Design review of the part built by this model. Coordinates are the model's own, in mm. Face numbers are marked on the shaded views. A direction names the side the tool comes from. Give positions to 0.01 mm unless a question says otherwise; leave off trailing zeros. Loops run counter-clockwise (first coordinate to the right, second up) from the corner with the lowest first, then second, coordinate; pieces in that order, holes last. Notation, with made-up numbers: M 65.25,-4 L 95.25,-4 A30 cw 95.25,32 Z; hole C -5.5,-2.75 d11. An arc over 180 degrees is marked long. Use a Markdown table: item, result. Add a question column.
(1) For the marked faces 4, 5 and 6, list the 3-axis set-ups (+Z, -Z, +X, -X, +Y, -Y) from which the entire face can be reached by the end or side of a thin tool; tool diameter is ignored.
(2) Add section A-A, the plane z = 27.5. Give the boundary of the cut face in (x, y).
(3) Add section C-C, the plane x = 86.5. Give the boundary of the cut face in (y, z).
(4) Add section D-D, the plane z = 16. Give the boundary of the cut face in (x, y).
(5) Insertion check: pin 1 Ø5 at (y, z) = (10, 14) entering from -X; pin 2 Ø10 at (x, z) = (24.5, 18) entering from -Y; pin 3 Ø5 at (x, z) = (34.92, 23.24) entering from +Y; pin 4 Ø1.9 at (y, z) = (11, 8) entering from +X. Each pin has a flat end and moves straight along its axis. Give the tip position at first contact, or say it passes through.
(6) For probe 1 along X at (y, z) = (7, 2); probe 2 along X at (y, z) = (9, 18.5); probe 3 along X at (y, z) = (7.5, 7.5), list the stretches that pass through material, from the lowest coordinate up.
(7) Add section B-B, the plane y = 9.5. State how many separate pieces and enclosed holes the cut face has, then the cut area to 3 significant figures.
(8) Draft analysis for pull direction Z (two halves, no side actions). For the marked faces 1, 2 and 3, state which applies: pulls with the +Z half, pulls with the -Z half, needs draft (parallel to the pull), parting line crosses it, or undercut.
```python
from build123d import *

# Parameters (mm, degrees)
F0_W      = 12.7
F0_H      = 31.75
F1_DEPTH  = 139.7
F2_W      = 12.7
F2_H      = 6.35
F2_W_2    = 6.35
F3_DEPTH  = 31.751
F4_R      = 2.159
F5_DEPTH  = 25.4
F6_R      = 2.159
F7_DEPTH  = 25.4
F8_W      = 50.8
F8_H      = 19.05
F9_DEPTH  = 6.35
F10_W     = 6.35
F10_H     = 19.05
F11_DEPTH = 6.35
F12_R     = 3.17499


# Not quite as in the source:
# - a fillet or chamfer is up to 0.001 mm smaller than in the source, because OpenCascade refuses the exact size


with BuildPart() as f1:
    # F0 (on Right) → F1 (new body)
    with BuildSketch(Plane.YZ):
        with Locations((6.35, 15.875)):
            Rectangle(F0_W, F0_H)
    extrude(amount=F1_DEPTH)

    # F2 (on face) → F3 (cut, through all)
    with BuildSketch(Plane.XY.offset(31.75)):
        with Locations((6.35, 9.525)):
            Rectangle(F2_W, F2_H)
        with Locations((34.925, 9.525)):
            Rectangle(F2_W_2, F2_H)
        with Locations((104.775, 9.525)):
            Rectangle(F2_W_2, F2_H)
        with Locations((133.35, 9.525)):
            Rectangle(F2_W, F2_H)
    extrude(amount=-F3_DEPTH, mode=Mode.SUBTRACT)

    # F4 (on face) → F5 (cut)
    with BuildSketch(Plane.XZ):
        with Locations((6.3445889391, 23.241)):
            Circle(F4_R)
        with Locations((6.3445889391, 8.509)):
            Circle(F4_R)
        with BuildLine():
            ThreePointArc((135.5180395808, 8.509), (133.3590395808, 10.668), (131.2000395808, 8.509))
            ThreePointArc((131.2000395808, 8.509), (133.3590395808, 6.35), (135.5180395808, 8.509))
        make_face()
        with BuildLine():
            ThreePointArc((135.5180395808, 23.241), (133.3590395808, 25.4), (131.2000395808, 23.241))
            ThreePointArc((131.2000395808, 23.241), (133.3590395808, 21.082), (135.5180395808, 23.241))
        make_face()
    extrude(amount=-F5_DEPTH, mode=Mode.SUBTRACT)

    # F6 (on face) → F7 (cut)
    with BuildSketch(Plane.XZ):
        with Locations((34.9172241986, 23.241)):
            Circle(F6_R)
        with Locations((34.9172241986, 8.509)):
            Circle(F6_R)
        with Locations((104.6765521169, 8.509)):
            Circle(F6_R)
        with Locations((104.6765521169, 23.241)):
            Circle(F6_R)
    extrude(amount=-F7_DEPTH, mode=Mode.SUBTRACT)

    # F8 (on face) → F9 (cut)
    with BuildSketch(Plane(origin=(0, 12.7, 0), x_dir=(-1, 0, 0), z_dir=(0, 1, 0))):
        with Locations((-69.85, 15.875)):
            Rectangle(F8_W, F8_H)
    extrude(amount=-F9_DEPTH, mode=Mode.SUBTRACT)

    # F10 (on face) → F11 (cut)
    with BuildSketch(Plane(origin=(0, 12.7, 0), x_dir=(-1, 0, 0), z_dir=(0, 1, 0))):
        with Locations((-22.225, 15.875)):
            Rectangle(F10_W, F10_H)
        with Locations((-117.475, 15.875)):
            Rectangle(F10_W, F10_H)
    extrude(amount=-F11_DEPTH, mode=Mode.SUBTRACT)

    # F12 (radius 3.175 in the source; OpenCascade refuses exactly that, so slightly less here)
    f12_edges = [f1.edges().sort_by_distance(p)[0] for p in [
        (19.05, 9.525, 6.35),
        (25.4, 9.525, 6.35),
        (19.05, 9.525, 25.4),
        (25.4, 9.525, 25.4),
        (44.45, 9.525, 6.35),
        (95.25, 9.525, 6.35),
        (95.25, 9.525, 25.4),
        (44.45, 9.525, 25.4),
        (120.65, 9.525, 6.35),
        (120.65, 9.525, 25.4),
        (114.3, 9.525, 25.4),
        (114.3, 9.525, 6.35),
    ]]
    fillet(f12_edges, radius=F12_R)


solid = f1.part
```
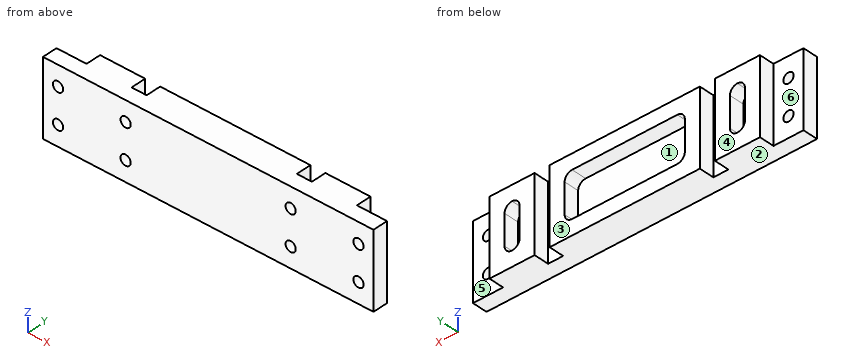
Established:
| question | item | result |
|---|---|---|
| 1 | face 4 | +Z, -Z, +X, -X, +Y |
| 1 | face 5 | +Z, -Z, +X, +Y |
| 1 | face 6 | +Z, -Z, -X, +Y |
| 2 | outline | M 0,0 L 139.7,0 L 139.7,6.35 L 127,6.35 L 127,12.7 L 107.95,12.7 L 107.95,6.35 L 101.6,6.35 L 101.6,12.7 L 38.1,12.7 L 38.1,6.35 L 31.75,6.35 L 31.75,12.7 L 12.7,12.7 L 12.7,6.35 L 0,6.35 Z |
| 3 | outline | M 0,0 L 12.7,0 L 12.7,6.35 L 6.35,6.35 L 6.35,25.4 L 12.7,25.4 L 12.7,31.75 L 0,31.75 Z |
| 4 | outline | M 0,0 L 139.7,0 L 139.7,6.35 L 127,6.35 L 127,12.7 L 120.65,12.7 L 120.65,6.35 L 114.3,6.35 L 114.3,12.7 L 107.95,12.7 L 107.95,6.35 L 101.6,6.35 L 101.6,12.7 L 95.25,12.7 L 95.25,6.35 L 44.45,6.35 L 44.45,12.7 L 38.1,12.7 L 38.1,6.35 L 31.75,6.35 L 31.75,12.7 L 25.4,12.7 L 25.4,6.35 L 19.05,6.35 L 19.05,12.7 L 12.7,12.7 L 12.7,6.35 L 0,6.35 Z |
| 5 | pin 1 | x = 12.7 |
| 5 | pin 2 | y = 0 |
| 5 | pin 3 | y = 6.35 |
| 5 | pin 4 | x = 127 |
| 6 | probe 1 | 12.7 to 31.75, 38.1 to 101.6, 107.95 to 127 |
| 6 | probe 2 | 12.7 to 19.05, 25.4 to 31.75, 38.1 to 44.45, 95.25 to 101.6, 107.95 to 114.3, 120.65 to 127 |
| 6 | probe 3 | 12.7 to 19.78, 24.67 to 31.75, 38.1 to 45.18, 94.52 to 101.6, 107.95 to 115.03, 119.92 to 127 |
| 7 | separate pieces | 3 |
| 7 | enclosed holes | 3 |
| 7 | area | 2,040 mm^2 |
| 8 | face 1 | undercut |
| 8 | face 2 | pulls with the -Z half |
| 8 | face 3 | needs draft |
